```python
from build123d import *

# Parameters (mm, degrees)
ESBO_O2_W                                 = 100
ESBO_O2_H                                 = 60
RESSALTO_EXTRUS_O1_DEPTH                  = 50
FURO1_D                                   = 14
FURO1_DEPTH                               = 9
FURO1_CBORE_D                             = 20
FURO1_CBORE_DEPTH                         = 3
FURO1_TIP                                 = 7
FURO2_D                                   = 16
FURO2_DEPTH                               = 11.193115048
FURO2_CSINK_D                             = 24
FURO2_CSINK_ANGLE                         = 90
FURO2_TIP                                 = 4.806884952
BROCA_DE_ROSQUEAR_PARA_TARRAXA_DE_M16X2_D = 14


with BuildPart() as part:
    # Esboço2 → Ressalto-extrusão1 (new body)
    with BuildSketch(Plane(origin=(0, 0, 0), x_dir=(1, 0, 0), z_dir=(0, 1, 0))):
        with Locations((-50, 30)):
            Rectangle(ESBO_O2_W, ESBO_O2_H)
    extrude(amount=RESSALTO_EXTRUS_O1_DEPTH)

    # Furo1
    with Locations(Plane(origin=(0, 50, 0), x_dir=(1, 0, 0), z_dir=(0, 1, 0))):
        with Locations((-50, 30)):
            CounterBoreHole(FURO1_D / 2, FURO1_CBORE_D / 2, FURO1_CBORE_DEPTH, depth=FURO1_DEPTH)
            with Locations((0, 0, -(FURO1_DEPTH + FURO1_TIP / 2))):  # 90° drill point
                Cone(0, FURO1_D / 2, FURO1_TIP, mode=Mode.SUBTRACT)

    # Furo2
    with Locations(Plane(origin=(0, 50, 0), x_dir=(1, 0, 0), z_dir=(0, 1, 0))):
        with Locations((-20, 30)):
            CounterSinkHole(FURO2_D / 2, FURO2_CSINK_D / 2, depth=FURO2_DEPTH, counter_sink_angle=FURO2_CSINK_ANGLE)
            with Locations((0, 0, -(FURO2_DEPTH + FURO2_TIP / 2))):  # 118° drill point
                Cone(0, FURO2_D / 2, FURO2_TIP, mode=Mode.SUBTRACT)

    # Broca de rosquear para tarraxa de M16x2.02 (through all)
    with Locations(Plane(origin=(0, 50, 0), x_dir=(1, 0, 0), z_dir=(0, 1, 0))):
        with Locations((-80, 30)):
            Hole(BROCA_DE_ROSQUEAR_PARA_TARRAXA_DE_M16X2_D / 2)


solid = part.part
```
For this review, take the finished solid that the model builds, in its own axes (mm). A direction names the side the tool comes from. Round coordinates to 2 decimals unless told otherwise and drop trailing zeros. Loops run counter-clockwise (first coordinate to the right, second up) from the corner with the lowest first, then second, coordinate; pieces in that order, holes last.
(1) We need section B-B (y = 44). Give the boundary of the cut face in (x, z).
Returned:
outline: (-100, -60) - (0, -60) - (0, 0) - (-100, 0) - close; hole circle Ø14 at (-80, -30); hole circle Ø14 at (-50, -30); hole circle Ø16 at (-20, -30)
(2) Tool access review of faces 4 (the cylindrical face through (-58, 49, -24)), 5 (the flat face through (0, 25, -30)): name each direction out of +Z, -Z, +X, -X, +Y, -Y from which nothing blocks a thin tool from reaching the whole face with its end or side.
Returned:
face 4: +Y
face 5: +Z, -Z, +X, +Y, -Y
(3) We need section A-A (x = -80). Give the boundary of the cut face in (y, z), plus the area to 3 significant figures.
Returned:
outline: (0, -60) - (50, -60) - (50, -37) - (0, -37) - close; (0, -23) - (50, -23) - (50, 0) - (0, 0) - close
area: 2,300 mm2
(4) Wall thickness on line 1 along Z through (x, y) = (-50, 48); line 2 along Z through (x, y) = (-80, 25); line 3 along X through (y, z) = (28, -30): over which ranges is each line inside the solid? List them lowest first.
Returned:
line 1: z = -60 to -40, -20 to 0
line 2: z = -60 to -37, -23 to 0
line 3: x = -100 to -87, -73 to 0
(5) We need section C-C (y = 29.5). Give the boundary of the cut face in (x, z).
Returned:
outline: (-100, -60) - (0, -60) - (0, 0) - (-100, 0) - close; hole circle Ø14 at (-80, -30)
(6) Mouldability with a two-part tool opening along Z and no side actions: class faces 1 (the flat face through (-57, 47, -28)), 2 (the flat face through (-62, 50, -30)), 3 (the flat face through (-51, 25, -60)) as released by +Z, released by -Z, zero draft, split by the parting line, or undercut.
Returned:
face 1: undercut
face 2: zero draft
face 3: released by -Z
(7) Clearance check with a flat-ended pin moving along its axis: P1, Ø16, axis at x = -51.5, z = -29, coming from the +Y side. State where the tip first meets the part, or that it passes through.
Returned:
P1: stops at y = 47
